Geometry: final body of the model. Coordinates: model frame, mm. Round coordinates to 2 decimals unless told otherwise and drop trailing zeros. Loops run counter-clockwise (first coordinate to the right, second up) from the corner with the lowest first, then second, coordinate; pieces in that order, holes last. Notation, with made-up numbers: (-25, 59) - (15, 59) arc R17 cw to (15, 68) - close; hole circle Ø5 at (48, -17.5). An arc over 180 degrees is marked (long way). Answer as a JSON object with one key per item and string values. Group by question number.
Item 1: Line query: line 1 (Y direction, x = 2, z = 80); line 2 (X direction, y = 0, z = -106.5); line 3 (Z direction, x = 27, y = 11.5). Output: solid intervals per line, ascending.
Item 2: Draft query along Y for faces 1 (the face through (-63.36, -14.17, -104.94)), 2 (the face through (35, -1, 35)), 3 (the face through (-54, 1, -100)), 4 (the face through (6, -40, 10)). Return one class per face: released by +Y, released by -Y, zero draft, split by the parting line, or undercut.
Item 3: Section D-D (x = 47). Return the cut outline in (y, z) (3 decimals).
Item 4: Section B-B (z = -29). Return the cut outline in (x, y).
Item 5: First-contact query: pin 1 (4.5 mm diameter, centred on y = 20, z = 80, fed in from +X); pin 2 (2.5 mm diameter, centred on x = 25.9, y = 24.5, fed in from +Z); pin 3 (4.5 mm diameter, centred on x = -14.02, y = 15, fed in from +Z) (3 decimals); pin 4 (1.8 mm diameter, centred on x = 16, y = 24.5, fed in from -Z). Flat tips, straight axial feed; report the tip coordinate or a pass-through.
Item 6: Section A-A (y = 0). Count the separate pieces of the cut face and the enclosed holes in it, plus the area to 3 significant figures.
Item 7: Section C-C (x = 30). Return the cut outline in (y, z).
```python
from build123d import *

# Parameters (mm, degrees)
SKETCH_1_W           = 200
SKETCH_1_H           = 80
EXTRUDE_1_DEPTH      = 10
SKETCH_2_W           = 10
SKETCH_2_H           = 80
EXTRUDE_2_DEPTH      = 50
SKETCH_3_W           = 100
SKETCH_3_H           = 100
EXTRUDE_3_DEPTH      = 10
EXTRUDE_4_DEPTH      = 15
EXTRUDE_5_DEPTH      = 15
FILLET_1_R           = 20
SKETCH_7_R           = 2.75
CUT_EXTRUDE_1_DEPTH  = 15
CUT_EXTRUDE_START    = -60
SKETCH_8_R           = 1.5
CUT_EXTRUDE_2_DEPTH  = 15
SKETCH_9_R           = 1.5
CUT_EXTRUDE_3_DEPTH  = 15
FILLET_2_R           = 20
SKETCH_16_R          = 2.75
CUT_EXTRUDE_7_DEPTH  = 225.944437584
CHAMFER_2_SIZE       = 0.5
CHAMFER_3_SIZE       = 0.5
EXTRUDE_8_DEPTH      = 10
CUT_EXTRUDE_8_DEPTH  = 225.944437584
CUT_EXTRUDE_9_DEPTH  = 225.944437584
SKETCH_20_R          = 2
CUT_EXTRUDE_10_DEPTH = 151.665191733
FILLET_3_R           = 10


with BuildPart() as part:
    # 草图1 → 凸台-拉伸1 (new body)
    with BuildSketch(Plane(origin=(0, 0, 0), x_dir=(0, 0, -1), z_dir=(1, 0, 0))):
        Rectangle(SKETCH_1_W, SKETCH_1_H)
    extrude(amount=EXTRUDE_1_DEPTH)

    # 草图2 → 凸台-拉伸2 (add)
    with BuildSketch(Plane(origin=(10, 0, 0), x_dir=(0, 0, -1), z_dir=(1, 0, 0))):
        with Locations((-30, 0)):
            Rectangle(SKETCH_2_W, SKETCH_2_H)
        with Locations((30, 0)):
            Rectangle(SKETCH_2_W, SKETCH_2_H)
    extrude(amount=EXTRUDE_2_DEPTH)

    # 草图3 → 凸台-拉伸3 (add)
    with BuildSketch(Plane(origin=(0, 0, -100), x_dir=(-1, 0, 0), z_dir=(0, 0, -1))):
        with Locations((40, 0)):
            Rectangle(SKETCH_3_W, SKETCH_3_H)
    extrude(amount=EXTRUDE_3_DEPTH)

    # 草图5 → 凸台-拉伸4 (add)
    with BuildSketch(Plane(origin=(0, 40, 0), x_dir=(1, 0, 0), z_dir=(0, 1, 0))):
        Polygon((10, 55), (-15, 100), (10, 100), align=None)
    extrude(amount=-EXTRUDE_4_DEPTH)

    # 草图6 → 凸台-拉伸5 (add)
    with BuildSketch(Plane.XZ.offset(40)):
        Polygon((-15, -100), (0, -100), (0, -73), align=None)
    extrude(amount=-EXTRUDE_5_DEPTH)

    # 圆角1
    fillet_1_edges = [part.edges().sort_by_distance(p)[0] for p in [
        (10, 50, -105),
        (10, -50, -105),
        (-90, 50, -105),
        (-90, -50, -105),
    ]]
    fillet(fillet_1_edges, radius=FILLET_1_R)

    # 草图7 → 切除-拉伸1 (cut)
    with BuildSketch(Plane(origin=(0, 0, -110), x_dir=(-1, 0, 0), z_dir=(0, 0, -1))):
        with Locations(Location((40, 30, 0), (0, 0, 90))):
            Circle(SKETCH_7_R)
        with Locations(Location((10, 0, 0), (0, 0, 90))):
            Circle(SKETCH_7_R)
        with Locations(Location((70, 0, 0), (0, 0, 90))):
            Circle(SKETCH_7_R)
        with Locations(Location((40, -30, 0), (0, 0, 90))):
            Circle(SKETCH_7_R)
    extrude(amount=-CUT_EXTRUDE_1_DEPTH, mode=Mode.SUBTRACT)

    # 草图8 → 切除-拉伸2 (cut)
    with BuildSketch(Plane(origin=(0, 0, -35), x_dir=(-1, 0, 0), z_dir=(0, 0, -1)).offset(CUT_EXTRUDE_START)):
        with Locations(Location((-16, 24.5, 0), (0, 0, 90))):
            Circle(SKETCH_8_R)
        with Locations(Location((-25.9, 24.5, 0), (0, 0, 90))):
            Circle(SKETCH_8_R)
        with Locations(Location((-16, -24.5, 0), (0, 0, 90))):
            Circle(SKETCH_8_R)
        with Locations(Location((-25.9, -24.5, 0), (0, 0, 90))):
            Circle(SKETCH_8_R)
    extrude(amount=-CUT_EXTRUDE_2_DEPTH, mode=Mode.SUBTRACT)

    # 草图9 → 切除-拉伸3 (cut)
    with BuildSketch(Plane.XY.offset(35).offset(CUT_EXTRUDE_START)):
        with Locations((21.5, 12)):
            Circle(SKETCH_9_R)
        with Locations((21.5, -12)):
            Circle(SKETCH_9_R)
    extrude(amount=-CUT_EXTRUDE_3_DEPTH, mode=Mode.SUBTRACT)

    # 圆角2
    fillet_2_edges = [part.edges().sort_by_distance(p)[0] for p in [
        (60, -40, 30),
        (60, 40, 30),
        (60, -40, -30),
        (60, 40, -30),
    ]]
    fillet(fillet_2_edges, radius=FILLET_2_R)

    # 草图16 → 切除-拉伸7 (cut, through all)
    with BuildSketch(Plane.XY.offset(-100)):
        with Locations((-25, 25.980762114)):
            Circle(SKETCH_16_R)
        with Locations((-14.019237886, 15)):
            Circle(SKETCH_16_R)
        with Locations(Location((-25, -25.980762114, 0), (0, 0, 180))):
            Circle(SKETCH_16_R)
        with Locations(Location((-14.019237886, -15, 0), (0, 0, 180))):
            Circle(SKETCH_16_R)
        with Locations(Location((-55, 25.980762114, 0), (0, 0, 180))):
            Circle(SKETCH_16_R)
        with Locations(Location((-65.980762114, 15, 0), (0, 0, 180))):
            Circle(SKETCH_16_R)
        with Locations((-55, -25.980762114)):
            Circle(SKETCH_16_R)
        with Locations((-65.980762114, -15)):
            Circle(SKETCH_16_R)
    extrude(amount=-CUT_EXTRUDE_7_DEPTH, mode=Mode.SUBTRACT)

    # 倒角2
    chamfer_2_edges = [part.edges().sort_by_distance(p)[0] for p in [
        (-70, -2.75, -100),
        (-70, -2.75, -110),
        (-40, -32.75, -100),
        (-40, -32.75, -110),
        (-52.25, 25.980762114, -110),
        (-52.25, 25.980762114, -100),
        (-68.730762114, -15, -110),
        (-68.730762114, -15, -100),
        (-57.75, -25.980762114, -110),
        (-57.75, -25.980762114, -100),
        (-63.230762114, 15, -110),
        (-63.230762114, 15, -100),
    ]]
    chamfer(chamfer_2_edges, length=CHAMFER_2_SIZE)

    # 倒角3
    chamfer_3_edges = [part.edges().sort_by_distance(p)[0] for p in [
        (-40, 27.25, -100),
        (-40, 27.25, -110),
        (-10, -2.75, -100),
        (-10, -2.75, -110),
        (-11.269237886, -15, -110),
        (-11.269237886, -15, -100),
        (-22.25, -25.980762114, -110),
        (-22.25, -25.980762114, -100),
        (-16.769237886, 15, -110),
        (-16.769237886, 15, -100),
        (-27.75, 25.980762114, -110),
        (-27.75, 25.980762114, -100),
    ]]
    chamfer(chamfer_3_edges, length=CHAMFER_3_SIZE)

    # 草图17 → 凸台-拉伸8 (add)
    with BuildSketch(Plane.XZ.offset(40)):
        Polygon((7.320508076, -100), (-40, -100), (7.320508076, -67.5), align=None)
    extrude_8 = extrude(amount=EXTRUDE_8_DEPTH)

    # 草图18 → 切除-拉伸8 (cut, through all)
    with BuildSketch(Plane(origin=(0, 0, -100), x_dir=(-1, 0, 0), z_dir=(0, 0, -1))):
        with BuildLine():
            Line((-7.320508076, -40), (-7.320508076, -50))
            Line((-7.320508076, -50), (10, -50))
            ThreePointArc((10, -50), (0, -47.320508076), (-7.320508076, -40))
        make_face()
    extrude(amount=-CUT_EXTRUDE_8_DEPTH, mode=Mode.SUBTRACT)

    # 镜向2: 凸台-拉伸8 across plane
    add(extrude_8.mirror(Plane.ZX))

    # 草图19 → 切除-拉伸9 (cut, through all)
    with BuildSketch(Plane(origin=(0, 0, -100), x_dir=(-1, 0, 0), z_dir=(0, 0, -1))):
        with BuildLine():
            Line((-7.320508076, 50), (-7.320508076, 40))
            ThreePointArc((-7.320508076, 40), (0, 47.320508076), (10, 50))
            Line((10, 50), (-7.320508076, 50))
        make_face()
    extrude(amount=-CUT_EXTRUDE_9_DEPTH, mode=Mode.SUBTRACT)

    # 草图20 → 切除-拉伸10 (cut, through all)
    with BuildSketch(Plane.ZY):
        with Locations((80, 20)):
            Circle(SKETCH_20_R)
        with Locations((80, -20)):
            Circle(SKETCH_20_R)
        with Locations((-60, 20)):
            Circle(SKETCH_20_R)
        with Locations((-60, -20)):
            Circle(SKETCH_20_R)
    extrude(amount=-CUT_EXTRUDE_10_DEPTH, mode=Mode.SUBTRACT)

    # 圆角3
    fillet_3_edges = [part.edges().sort_by_distance(p)[0] for p in [
        (5, 40, 100),
        (5, -40, 100),
    ]]
    fillet(fillet_3_edges, radius=FILLET_3_R)


solid = part.part
```
Values:
{
 "1": {"line 1": "y = -40 to -22, -18 to 18, 22 to 40", "line 2": "x = -90 to -72.75, -67.25 to -12.75, -7.25 to 10", "line 3": "z = -35 to -25, 25 to 35"},
 "2": {"face 1": "undercut", "face 2": "zero draft", "face 3": "undercut", "face 4": "released by -Y"},
 "3": {"outline": "(-38.735, -35) - (38.735, -35) - (38.735, -25) - (-38.735, -25) - close; (-38.735, 25) - (38.735, 25) - (38.735, 35) - (-38.735, 35) - close"},
 "4": {"outline": "(0, -40) - (40, -40) arc R20 ccw to (60, -20) - (60, 20) arc R20 ccw to (40, 40) - (0, 40) - close; hole circle Ø3 at (21.5, -12); hole circle Ø3 at (21.5, 12)"},
 "5": {"pin 1": "stops at x = 10", "pin 2": "stops at z = -25", "pin 3": "passes through", "pin 4": "stops at z = -35"},
 "6": {"separate pieces": "3", "enclosed holes": "0", "area": "3,890 mm^2"},
 "7": {"outline": "(-40, -35) - (40, -35) - (40, -25) - (-40, -25) - close; (-40, 25) - (40, 25) - (40, 35) - (-40, 35) - close"}
}
